Part model, mm, in its own coordinate system. Face numbers are marked on the shaded views. A direction names the side the tool comes from. Coordinates: 2 decimals unless noted, no trailing zeros. Write each loop counter-clockwise with the first axis right and the second up, starting at its lowest first coordinate (ties: lowest second). Pieces come first, ordered by that corner, then holes. Notation, with made-up numbers: (5.25, 70.25) -> (22.25, 70.25) arc R21 cw to (22.25, 84.25) -> close; hole circle Ø4 at (14.5, -21.5). An arc over 180 degrees is marked (long way). Write item = value, one per line.
from build123d import *

# Parameters (mm, degrees)
ESQUISSE1_W                         = 32.5
ESQUISSE1_H                         = 42.5
ESQUISSE2_W                         = 9
ESQUISSE2_H                         = 58.5
CONG_R2_R                           = 2
ESQUISSE3_W                         = 4
ESQUISSE3_H                         = 0.25
D_GROSSISEMENT_OUTLINE_R            = 42.5
D_GROSSISEMENT_OUTLINE_W            = 22.5
D_GROSSISEMENT_OUTLINE_H            = 79
D_GROSSISEMENT_DEPTH                = 15.5
FINITION_EXT_R                      = 11.25
USINAGE_EN_V_DEPTH                  = 63.461988441
USINAGE_EN_V_DEPTH_BACK             = 63.461988441
RAINURE_INT_DEPTH                   = 63.461988441
ESQUISSE10_W                        = 2.5
ESQUISSE10_H                        = 15.5
TROU_TARAUD_M61_AT_2_COUNT          = 2
TROU_TARAUD_M61_AT_2_PITCH          = 62
TROU_TARAUD_M41_D                   = 3.3
DIAM_TRE_DU_PER_AGE_6_0_6_1_D       = 6
DIAM_TRE_DU_PER_AGE_2_5_2_5_1_D     = 2.5
DIAM_TRE_DU_PER_AGE_2_5_2_5_1_DEPTH = 3
DIAM_TRE_DU_PER_AGE_2_5_2_5_1_TIP   = 0.751075774


# Read off the part's stored shape, not the designer's step: Dégrossisement
with BuildPart() as part:
    # Esquisse1 → Brut (revolve)
    with BuildSketch(Plane.XY, mode=Mode.PRIVATE) as brut_sk:
        with Locations((-0.75, 21.25)):
            Rectangle(ESQUISSE1_W, ESQUISSE1_H)
    revolve(brut_sk.sketch.rotate(Axis((-714.885574261, 0, 0), (1, 0, 0)), 90), axis=Axis((-714.885574261, 0, 0), (1, 0, 0)))

    # Esquisse2 → Pion désaxer (revolve, cut)
    with BuildSketch(Plane.XY, mode=Mode.PRIVATE) as pion_d_saxer_sk:
        with Locations((-12.5, -13.25)):
            Rectangle(ESQUISSE2_W, ESQUISSE2_H)
    revolve(pion_d_saxer_sk.sketch.rotate(Axis((-1017, 20.5, 0), (1, 0, 0)), 270), axis=Axis((-1017, 20.5, 0), (1, 0, 0)), mode=Mode.SUBTRACT)

    # Congé R2
    cong_r2_edges = [part.edges().sort_by_distance(p)[0] for p in [
        (-8, 20.5, -4.5),
    ]]
    fillet(cong_r2_edges, radius=CONG_R2_R)

    # Esquisse3 → Enlèv. Ø83d9 (revolve, cut)
    with BuildSketch(Plane.XY, mode=Mode.PRIVATE) as enl_v_83d9_sk:
        with Locations((-6, 42.375)):
            Rectangle(ESQUISSE3_W, ESQUISSE3_H)
    revolve(enl_v_83d9_sk.sketch.rotate(Axis((-1000, 0, 0), (1, 0, 0)), 90), axis=Axis((-1000, 0, 0), (1, 0, 0)), mode=Mode.SUBTRACT)

    # Dégrossisement outline → Dégrossisement (cut)
    with BuildSketch(Plane(origin=(0, 0, 0), x_dir=(0, 0, -1), z_dir=(1, 0, 0))):
        Circle(D_GROSSISEMENT_OUTLINE_R)
        Rectangle(D_GROSSISEMENT_OUTLINE_W, D_GROSSISEMENT_OUTLINE_H, mode=Mode.SUBTRACT)
    extrude(amount=D_GROSSISEMENT_DEPTH, mode=Mode.SUBTRACT)

    # Finition ext.
    finition_ext_edges = [part.edges().sort_by_distance(p)[0] for p in [
        (7.75, -39.5, -11.25),
        (7.75, -39.5, 11.25),
        (7.75, 39.5, -11.25),
        (7.75, 39.5, 11.25),
    ]]
    fillet(finition_ext_edges, radius=FINITION_EXT_R - 0.0001)  # a hair under: the kernel refuses the full size

    # Esquisse5 → Usinage en V (cut, two sides: drawn at the far end of the back side and taken through both)
    with BuildSketch(Plane.XY.offset(-USINAGE_EN_V_DEPTH_BACK)):
        Polygon((0, -9.05), (0, 9.05), (15.5, 17.998929172), (15.5, -17.998929172), align=None)
    extrude(amount=USINAGE_EN_V_DEPTH + USINAGE_EN_V_DEPTH_BACK, mode=Mode.SUBTRACT)

    # Esquisse6 → Rainure Int. (cut, through all)
    with BuildSketch(Plane(origin=(0, 0, 0), x_dir=(0, 0, -1), z_dir=(1, 0, 0))):
        with BuildLine():
            Line((7, 20.5), (7, -20.5))
            ThreePointArc((7, -20.5), (0, -27.5), (-7, -20.5))
            Line((-7, -20.5), (-7, 20.5))
            ThreePointArc((-7, 20.5), (0, 27.5), (7, 20.5))
        make_face()
    extrude(amount=RAINURE_INT_DEPTH, mode=Mode.SUBTRACT)

    # Esquisse10 → Trou taraudé M61 (revolve, cut)
    with BuildSketch(Plane.ZX.offset(31)):
        with Locations((1.25, 7.75)):
            Rectangle(ESQUISSE10_W, ESQUISSE10_H)
    trou_taraud_m61 = revolve(axis=Axis((-6.35, 31, 0), (1, 0, 0)), mode=Mode.SUBTRACT)

    # Trou taraudé M61 at 2: Trou taraudé M61 ×2
    with Locations(*[(0, -i * TROU_TARAUD_M61_AT_2_PITCH, 0) for i in range(1, TROU_TARAUD_M61_AT_2_COUNT)]):
        add(trou_taraud_m61, mode=Mode.SUBTRACT)

    # Trou taraudé M41 (through all)
    with Locations(Plane.ZY.offset(17)):
        with Locations((0, 20.5)):
            Hole(TROU_TARAUD_M41_D / 2)

    # Diamètre du perçage Ø6.0 (6)1 (through all)
    with Locations(Plane.ZY.offset(8)):
        with Locations((-21, -29)):
            Hole(DIAM_TRE_DU_PER_AGE_6_0_6_1_D / 2)

    # Diamètre du perçage Ø2.5 (2.5)1
    with Locations(Plane(origin=(-5.25, 42.25, 0), x_dir=(0, 0, 1), z_dir=(0, 1, 0))):
        with Locations((0, 0)):
            Hole(DIAM_TRE_DU_PER_AGE_2_5_2_5_1_D / 2, depth=DIAM_TRE_DU_PER_AGE_2_5_2_5_1_DEPTH)
            with Locations((0, 0, -(DIAM_TRE_DU_PER_AGE_2_5_2_5_1_DEPTH + DIAM_TRE_DU_PER_AGE_2_5_2_5_1_TIP / 2))):  # 118° drill point
                Cone(0, DIAM_TRE_DU_PER_AGE_2_5_2_5_1_D / 2, DIAM_TRE_DU_PER_AGE_2_5_2_5_1_TIP, mode=Mode.SUBTRACT)


solid = part.part
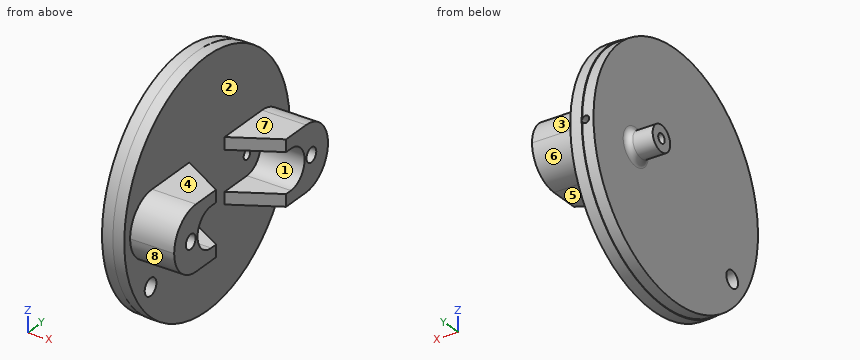
Q1. Which spindle directions (+Z, -Z, +X, -X, +Y, -Y) get a long thin tool onto all of the face, cutting with end or side? Do the marked faces 5, 6, 7 and 8. Say none if no direction does.
Model answer:
face_5 = -Z, +X, +Y, -Y
face_6 = -Z, +X, +Y
face_7 = +Z, +X, +Y, -Y
face_8 = -Z, +X, -Y
Q2. Mould opens along Y. For the marked faces 1, 2, 3 and 4 say: released by +Y, released by -Y, zero draft, split by the parting line, or undercut.
Model answer:
face_1 = undercut
face_2 = undercut
face_3 = released by +Y
face_4 = zero draft
Q3. Pin check, flat tips, straight feed: pin 1 (1.5 mm diameter, centred on x = 9.5, z = 11, fed in from +Y); pin 2 (4.5 mm diameter, centred on x = 10, y = -18, fed in from -Z); pin 3 (6 mm diameter, centred on y = 28.5, z = 27.5, fed in from -X); pin 4 (3.5 mm diameter, centred on y = -29, z = -21, fed in from -X). Stop position of each tip, or through.
Model answer:
pin_1 = 32.89
pin_2 = -11.25
pin_3 = -8
pin_4 = through
Q4. Saw through at B-B on z = -9.5. Give the cut face in (x, y), and give its area (3 significant figures).
Model answer:
outline = (-8, -41.17) -> (-4, -41.17) -> (-4, -41.42) -> (0, -41.42) -> (0, -34.28) -> (15.5, -34.28) -> (15.5, -18) -> (0, -9.05) -> (0, 9.05) -> (15.5, 18) -> (15.5, 34.28) -> (0, 34.28) -> (0, 41.42) -> (-4, 41.42) -> (-4, 41.17) -> (-8, 41.17) -> close
area = 1,300 mm²
Q5. Probe line 1 (Y direction, x = 8, z = 0); line 2 (Z direction, x = 13, y = -20.5); line 3 (Y direction, x = 6.5, z = -1). List the from-to ranges inside material, lowest first. Write a range as from..to.
Model answer:
line_1 = -39.5..-33.5, -28.5..-27.5, 27.5..28.5, 33.5..39.5
line_2 = -11.25..-7, 7..11.25
line_3 = -39.46..-33.29, -28.71..-27.43, 27.43..28.71, 33.29..39.46
Q6. Saw through at D-D on y = 31. Give the cut face in (x, z), and give its area (3 significant figures).
Model answer:
outline = (-8, -28.71) -> (-4, -28.71) -> (-4, -29.07) -> (0, -29.07) -> (0, -10.91) -> (15.5, -10.91) -> (15.5, -2.5) -> (0, -2.5) -> (0, 2.5) -> (15.5, 2.5) -> (15.5, 10.91) -> (0, 10.91) -> (0, 29.07) -> (-4, 29.07) -> (-4, 28.71) -> (-8, 28.71) -> close
area = 723 mm²
Q7. Saw through at C-C on x = -13.5. Give the cut face in (y, z), and give its area (3 significant figures).
Model answer:
outline = circle Ø9 at (20.5, 0); hole circle Ø3.3 at (20.5, 0)
area = 55.1 mm²
Q8. Saw through at A-A on x = 2. Count the separate pieces of the cut face and the enclosed holes in it, and give its area (3 significant figures).
Model answer:
separate_pieces = 2
enclosed_holes = 2
area = 728 mm²
